```python
from build123d import *

# Parameters (mm, degrees)
SKETCH_1_R          = 1.5
SKETCH_1_R_2        = 0.8
EXTRUDE_1_DEPTH     = 9.6
CUT_EXTRUDE_START   = -5.1
CUT_EXTRUDE_1_DEPTH = 5.1
SKETCH_3_W          = 90
SKETCH_3_H          = 57
CUT_EXTRUDE_2_DEPTH = 7.1
FILLET_1_R          = 3
FILLET_2_R          = 1
SKETCH_13_W         = 12
SKETCH_13_H         = 12
CUT_EXTRUDE_3_DEPTH = 73.118652234


with BuildPart() as part:
    # 草图1 → 凸台-拉伸1 (new body)
    with BuildSketch(Plane(origin=(0, 0, 0), x_dir=(1, 0, 0), z_dir=(0, 1, 0))):
        with BuildLine():
            Line((-47.5, 23), (-47.5, -23))
            ThreePointArc((-47.5, -23), (-48.085786438, -24.414213562), (-49.5, -25))
            Line((-49.5, -25), (-50.8, -25))
            ThreePointArc((-50.8, -25), (-53.8, -28), (-50.8, -31))
            Line((-50.8, -31), (-49.5, -31))
            ThreePointArc((-49.5, -31), (-48.085786438, -31.585786438), (-47.5, -33))
            Line((-47.5, -33), (-47.5, -44.5))
            ThreePointArc((-47.5, -44.5), (-46.621320344, -46.621320344), (-44.5, -47.5))
            Line((-44.5, -47.5), (-41.25, -47.5))
            Line((-41.25, -47.5), (-41.25, -34.5))
            Line((-41.25, -34.5), (-17.75, -34.5))
            Line((-17.75, -34.5), (-17.75, -47.5))
            Line((-17.75, -47.5), (-15.5, -47.5))
            ThreePointArc((-15.5, -47.5), (-13.378679656, -46.621320344), (-12.5, -44.5))
            Line((-12.5, -44.5), (-12.5, -33))
            ThreePointArc((-12.5, -33), (-11.914213562, -31.585786438), (-10.5, -31))
            Line((-10.5, -31), (-5, -31))
            ThreePointArc((-5, -31), (-3.585786438, -31.585786438), (-3, -33))
            Line((-3, -33), (-3, -33.8))
            ThreePointArc((-3, -33.8), (0, -36.8), (3, -33.8))
            Line((3, -33.8), (3, -33))
            ThreePointArc((3, -33), (3.585786438, -31.585786438), (5, -31))
            Line((5, -31), (10.5, -31))
            ThreePointArc((10.5, -31), (11.914213562, -31.585786438), (12.5, -33))
            Line((12.5, -33), (12.5, -44.5))
            ThreePointArc((12.5, -44.5), (13.378679656, -46.621320344), (15.5, -47.5))
            Line((15.5, -47.5), (17.75, -47.5))
            Line((17.75, -47.5), (17.75, -34.5))
            Line((17.75, -34.5), (41.25, -34.5))
            Line((41.25, -34.5), (41.25, -47.5))
            Line((41.25, -47.5), (44.5, -47.5))
            ThreePointArc((44.5, -47.5), (46.621320344, -46.621320344), (47.5, -44.5))
            Line((47.5, -44.5), (47.5, -33))
            ThreePointArc((47.5, -33), (48.085786438, -31.585786438), (49.5, -31))
            Line((49.5, -31), (50.8, -31))
            ThreePointArc((50.8, -31), (53.8, -28), (50.8, -25))
            Line((50.8, -25), (49.5, -25))
            ThreePointArc((49.5, -25), (48.085786438, -24.414213562), (47.5, -23))
            Line((47.5, -23), (47.5, 23))
            ThreePointArc((47.5, 23), (48.085786438, 24.414213562), (49.5, 25))
            Line((49.5, 25), (50.8, 25))
            ThreePointArc((50.8, 25), (53.8, 28), (50.8, 31))
            Line((50.8, 31), (49.5, 31))
            ThreePointArc((49.5, 31), (48.085786438, 31.585786438), (47.5, 33))
            Line((47.5, 33), (47.5, 44.5))
            ThreePointArc((47.5, 44.5), (46.621320344, 46.621320344), (44.5, 47.5))
            Line((44.5, 47.5), (41.25, 47.5))
            Line((41.25, 47.5), (41.25, 34.5))
            Line((41.25, 34.5), (17.75, 34.5))
            Line((17.75, 34.5), (17.75, 47.5))
            Line((17.75, 47.5), (15.5, 47.5))
            ThreePointArc((15.5, 47.5), (13.378679656, 46.621320344), (12.5, 44.5))
            Line((12.5, 44.5), (12.5, 33))
            ThreePointArc((12.5, 33), (11.914213562, 31.585786438), (10.5, 31))
            Line((10.5, 31), (5, 31))
            ThreePointArc((5, 31), (3.585786438, 31.585786438), (3, 33))
            Line((3, 33), (3, 33.8))
            ThreePointArc((3, 33.8), (0, 36.8), (-3, 33.8))
            Line((-3, 33.8), (-3, 33))
            ThreePointArc((-3, 33), (-3.585786438, 31.585786438), (-5, 31))
            Line((-5, 31), (-10.5, 31))
            ThreePointArc((-10.5, 31), (-11.914213562, 31.585786438), (-12.5, 33))
            Line((-12.5, 33), (-12.5, 44.5))
            ThreePointArc((-12.5, 44.5), (-13.378679656, 46.621320344), (-15.5, 47.5))
            Line((-15.5, 47.5), (-17.75, 47.5))
            Line((-17.75, 47.5), (-17.75, 34.5))
            Line((-17.75, 34.5), (-41.25, 34.5))
            Line((-41.25, 34.5), (-41.25, 47.5))
            Line((-41.25, 47.5), (-44.5, 47.5))
            ThreePointArc((-44.5, 47.5), (-46.621320344, 46.621320344), (-47.5, 44.5))
            Line((-47.5, 44.5), (-47.5, 33))
            ThreePointArc((-47.5, 33), (-48.085786438, 31.585786438), (-49.5, 31))
            Line((-49.5, 31), (-50.8, 31))
            ThreePointArc((-50.8, 31), (-53.8, 28), (-50.8, 25))
            Line((-50.8, 25), (-49.5, 25))
            ThreePointArc((-49.5, 25), (-48.085786438, 24.414213562), (-47.5, 23))
        make_face()
        with Locations(Location((-50.8, 28, 0), (0, 0, 270))):
            Circle(SKETCH_1_R, mode=Mode.SUBTRACT)
        with Locations(Location((50.8, 28, 0), (0, 0, 90))):
            Circle(SKETCH_1_R, mode=Mode.SUBTRACT)
        with Locations(Location((50.8, -28, 0), (0, 0, 270))):
            Circle(SKETCH_1_R, mode=Mode.SUBTRACT)
        with Locations(Location((-50.8, -28, 0), (0, 0, 90))):
            Circle(SKETCH_1_R, mode=Mode.SUBTRACT)
        with Locations(Location((0, 33.8, 0), (0, 0, 270))):
            Circle(SKETCH_1_R, mode=Mode.SUBTRACT)
        with Locations(Location((0, -33.8, 0), (0, 0, 90))):
            Circle(SKETCH_1_R, mode=Mode.SUBTRACT)
        with Locations(Location((43.5, 41, 0), (0, 0, 270))):
            Circle(SKETCH_1_R_2, mode=Mode.SUBTRACT)
        with Locations(Location((15.5, 41, 0), (0, 0, 90))):
            Circle(SKETCH_1_R_2, mode=Mode.SUBTRACT)
        with Locations(Location((43.5, -41, 0), (0, 0, 90))):
            Circle(SKETCH_1_R_2, mode=Mode.SUBTRACT)
        with Locations(Location((15.5, -41, 0), (0, 0, 270))):
            Circle(SKETCH_1_R_2, mode=Mode.SUBTRACT)
        with Locations(Location((-15.5, -41, 0), (0, 0, 90))):
            Circle(SKETCH_1_R_2, mode=Mode.SUBTRACT)
        with Locations(Location((-43.5, -41, 0), (0, 0, 270))):
            Circle(SKETCH_1_R_2, mode=Mode.SUBTRACT)
        with Locations(Location((-43.5, 41, 0), (0, 0, 90))):
            Circle(SKETCH_1_R_2, mode=Mode.SUBTRACT)
        with Locations(Location((-15.5, 41, 0), (0, 0, 270))):
            Circle(SKETCH_1_R_2, mode=Mode.SUBTRACT)
    extrude(amount=-EXTRUDE_1_DEPTH)

    # 草图2 → 切除-拉伸1 (cut)
    with BuildSketch(Plane.XZ.offset(9.6).offset(CUT_EXTRUDE_START)):
        with BuildLine():
            Line((63.557901373, 31), (5, 31))
            ThreePointArc((5, 31), (3.585786438, 31.585786438), (3, 33))
            Line((3, 33), (3, 33.8))
            ThreePointArc((3, 33.8), (0, 36.8), (-3, 33.8))
            Line((-3, 33.8), (-3, 33))
            ThreePointArc((-3, 33), (-3.585786438, 31.585786438), (-5, 31))
            Line((-5, 31), (-73.010332056, 31))
            Line((-73.010332056, 31), (-73.010332056, 53.694218021))
            Line((-73.010332056, 53.694218021), (63.557901373, 53.694218021))
            Line((63.557901373, 53.694218021), (63.557901373, 31))
        make_face()
        with BuildLine():
            Line((63.557901373, -31), (63.557901373, -53.694218021))
            Line((63.557901373, -53.694218021), (-73.010332056, -53.694218021))
            Line((-73.010332056, -53.694218021), (-73.010332056, -31))
            Line((-73.010332056, -31), (-5, -31))
            ThreePointArc((-5, -31), (-3.585786438, -31.585786438), (-3, -33))
            Line((-3, -33), (-3, -33.8))
            ThreePointArc((-3, -33.8), (0, -36.8), (3, -33.8))
            Line((3, -33.8), (3, -33))
            ThreePointArc((3, -33), (3.585786438, -31.585786438), (5, -31))
            Line((5, -31), (63.557901373, -31))
        make_face()
    extrude(amount=CUT_EXTRUDE_1_DEPTH, mode=Mode.SUBTRACT)

    # 草图3 → 切除-拉伸2 (cut)
    with BuildSketch(Plane.XZ.offset(9.6)):
        Rectangle(SKETCH_3_W, SKETCH_3_H)
    extrude(amount=-CUT_EXTRUDE_2_DEPTH, mode=Mode.SUBTRACT)

    # 圆角1
    fillet_1_edges = [part.edges().sort_by_distance(p)[0] for p in [
        (45, -6.05, 28.5),
        (45, -6.05, -28.5),
        (-45, -6.05, -28.5),
        (-45, -6.05, 28.5),
    ]]
    fillet(fillet_1_edges, radius=FILLET_1_R)

    # 圆角2
    fillet_2_edges = [part.edges().sort_by_distance(p)[0] for p in [
        (0, -2.5, -28.5),
        (-45, -2.5, 0),
        (45, -2.5, 0),
        (0, -2.5, 28.5),
        (44.121320344, -2.5, 27.621320344),
        (44.121320344, -2.5, -27.621320344),
        (-44.121320344, -2.5, 27.621320344),
        (-44.121320344, -2.5, -27.621320344),
    ]]
    fillet(fillet_2_edges, radius=FILLET_2_R)

    # 草图13 → 切除-拉伸3 (cut, through all)
    with BuildSketch(Plane.XZ.offset(2.5)):
        with Locations((-33, 18)):
            Rectangle(SKETCH_13_W, SKETCH_13_H)
        with Locations((-16.6, 18)):
            Rectangle(SKETCH_13_W, SKETCH_13_H)
        with Locations((-0.2, 18)):
            Rectangle(SKETCH_13_W, SKETCH_13_H)
        with Locations((16.2, 18)):
            Rectangle(SKETCH_13_W, SKETCH_13_H)
        with Locations((32.6, 18)):
            Rectangle(SKETCH_13_W, SKETCH_13_H)
        with Locations((-16.6, 0)):
            Rectangle(SKETCH_13_W, SKETCH_13_H)
        with Locations((-0.2, 0)):
            Rectangle(SKETCH_13_W, SKETCH_13_H)
        with Locations((16.2, 0)):
            Rectangle(SKETCH_13_W, SKETCH_13_H)
        with Locations((32.6, 0)):
            Rectangle(SKETCH_13_W, SKETCH_13_H)
        with Locations((-16.6, -18)):
            Rectangle(SKETCH_13_W, SKETCH_13_H)
        with Locations((-0.2, -18)):
            Rectangle(SKETCH_13_W, SKETCH_13_H)
        with Locations((16.2, -18)):
            Rectangle(SKETCH_13_W, SKETCH_13_H)
        with Locations((32.6, -18)):
            Rectangle(SKETCH_13_W, SKETCH_13_H)
        with Locations((-33, 0)):
            Rectangle(SKETCH_13_W, SKETCH_13_H)
        with Locations((-33, -18)):
            Rectangle(SKETCH_13_W, SKETCH_13_H)
    extrude(amount=-CUT_EXTRUDE_3_DEPTH, mode=Mode.SUBTRACT)


solid = part.part
```
CAD build for the part. Positions are in the model's coordinates, mm. A direction names the side the tool comes from. Round coordinates to 2 decimals unless told otherwise and drop trailing zeros. Write each loop counter-clockwise with the first axis right and the second up, starting at its lowest first coordinate (ties: lowest second). Pieces come first, ordered by that corner, then holes.
Item 1: Band-saw the part on A-A on z = 15. Give the number of separate pieces and of enclosed holes in the cut face, then the cut area to 3 significant figures.
Filled in:
separate pieces: 6
enclosed holes: 0
area: 123 mm2
Item 2: Drill centre lines: L1, parallel to X at y = -2.25, z = 3.5; L2, parallel to X at y = -2.5, z = 28; L3, parallel to Z at x = 43.5, y = -2. Where is each one in solid material? Low to high.
Filled in:
L1: x = -47.5 to -39, -27 to -22.6, -10.6 to -6.2, 5.8 to 10.2, 22.2 to 26.6, 38.6 to 47.5
L2: x = -53.8 to -52.3, -49.3 to 49.3, 52.3 to 53.8
L3: z = -47.5 to -41.8, -40.2 to 40.2, 41.8 to 47.5
Item 3: Mould opens along X. For faces 1 (the flat face through (-17, -2, 47.5)), 2 (the cylindrical face through (-44.14, -6.51, 27.6)), 3 (the cylindrical face through (53.8, -4.7, -27.9)) say: released by +X, released by -X, zero draft, split by the parting line, or undercut.
Filled in:
face 1: zero draft
face 2: undercut
face 3: released by +X
Item 4: Tool access for faces 4 (the flat face through (38.6, -1, 18)), 5 (the cylindrical face through (13.4, -2.22, -46.64)), 6 (the flat face through (-10, -2.5, 0)): list every direction of +Z, -Z, +X, -X, +Y, -Y with a clear straight run to the whole face (end or side of a thin tool).
Filled in:
face 4: +Y, -Y
face 5: -Z, +Y, -Y
face 6: -Y
Item 5: Drop flat-ended pins along their axis: pin 1 Ø1 at (x, y) = (50, -4) entering from +Z; pin 2 Ø5 at (x, z) = (34.5, 36.5) entering from -Y; pin 3 Ø1.5 at (y, z) = (-6.5, 22) entering from +X. Give the stop position or say it passes through.
Filled in:
pin 1: stops at z = 31
pin 2: stops at y = -4.5
pin 3: stops at x = 47.5
Item 6: Band-saw the part on B-B on x = 29. Write the cut outline in (y, z), then the cut area to 3 significant figures.
Filled in:
outline: (-9.6, -31) - (-4.5, -31) - (-4.5, -34.5) - (0, -34.5) - (0, -24) - (-2.5, -24) - (-2.5, -27.5) arc R1 cw to (-3.5, -28.5) - (-9.6, -28.5) - close; (-9.6, 28.5) - (-3.5, 28.5) arc R1 cw to (-2.5, 27.5) - (-2.5, 24) - (0, 24) - (0, 34.5) - (-4.5, 34.5) - (-4.5, 31) - (-9.6, 31) - close; (-2.5, -12) - (0, -12) - (0, -6) - (-2.5, -6) - close; (-2.5, 6) - (0, 6) - (0, 12) - (-2.5, 12) - close
area: 132 mm2
